Work out the finished part from the listing and answer in its coordinate system (mm). A direction names the side the tool comes from. Round coordinates to 2 decimals unless told otherwise and drop trailing zeros. Loops run counter-clockwise (first coordinate to the right, second up) from the corner with the lowest first, then second, coordinate; pieces in that order, holes last.
```python
from build123d import *

# Parameters (mm, degrees)
SKETCH1_W           = 20
SKETCH1_H           = 30
SKETCH1_R           = 2.65
BOSS_EXTRUDE1_DEPTH = 3
SKETCH2_W           = 20
SKETCH2_H           = 10
BOSS_EXTRUDE2_DEPTH = 3
SKETCH3_W           = 1.8
SKETCH3_H           = 10
BOSS_EXTRUDE3_DEPTH = 10
FILLET1_R           = 5
CUT_EXTRUDE1_REACH  = 29.78
SKETCH4_R           = 1.5
CHAMFER1_SIZE       = 2


with BuildPart() as part:
    # Sketch1 → Boss-Extrude1 (new body)
    with BuildSketch(Plane.XY):
        Rectangle(SKETCH1_W, SKETCH1_H)
        with Locations((0, -10)):
            Circle(SKETCH1_R, mode=Mode.SUBTRACT)
        Circle(SKETCH1_R, mode=Mode.SUBTRACT)
    extrude(amount=BOSS_EXTRUDE1_DEPTH)

    # Sketch2 → Boss-Extrude2 (add)
    with BuildSketch(Plane.XY.offset(3)):
        with Locations((0, 10)):
            Rectangle(SKETCH2_W, SKETCH2_H)
    extrude(amount=BOSS_EXTRUDE2_DEPTH)

    # Sketch3 → Boss-Extrude3 (add)
    with BuildSketch(Plane.XY.offset(6)):
        with Locations((-6.15, 10)):
            Rectangle(SKETCH3_W, SKETCH3_H)
        with Locations((6.15, 10)):
            Rectangle(SKETCH3_W, SKETCH3_H)
    extrude(amount=BOSS_EXTRUDE3_DEPTH)

    # Fillet1
    fillet1_edges = [part.edges().sort_by_distance(p)[0] for p in [
        (6.15, 5, 16),
        (-6.15, 5, 16),
        (6.15, 15, 16),
        (-6.15, 15, 16),
    ]]
    fillet(fillet1_edges, radius=FILLET1_R - 0.0001)  # a hair under: the kernel refuses the full size

    # Cut-Extrude1: up to this face of the body (flat: up to its plane)
    cut_extrude1_end = Plane(part.part.faces().sort_by_distance((7.05, 10, 10.533268934))[0])
    # Sketch4 → Cut-Extrude1 (cut, up to the picked face)
    with BuildSketch(Plane.ZY.offset(7.05), mode=Mode.PRIVATE) as cut_extrude1_sk1:
        with Locations(Location((11, 10, 0), (0, 0, 270))):
            Circle(SKETCH4_R)
    cut_extrude1_tool1 = split(extrude(cut_extrude1_sk1.sketch, amount=-CUT_EXTRUDE1_REACH, mode=Mode.PRIVATE), bisect_by=cut_extrude1_end, keep=Keep.BOTH, mode=Mode.PRIVATE)
    add(cut_extrude1_tool1.solids().sort_by(Axis((-7.05, 10, 11), (1, 0, 0)))[0], mode=Mode.SUBTRACT)

    # Chamfer1
    chamfer1_edges = [part.edges().sort_by_distance(p)[0] for p in [
        (-7.05, 10, 6),
        (7.05, 10, 6),
    ]]
    chamfer(chamfer1_edges, length=CHAMFER1_SIZE)


solid = part.part
```
1. Determine the mould class of faces 1 (the face through (-5.25, 8.8, 9.8)), 2 (the face through (0, 5, 5)), 3 (the face through (-0.57, -12.59, 1.48)) for opening direction Y: +Y half, -Y half, draft (parallel to the pull), parting line (faces both ways), or undercut.
Answer key:
face 1: draft
face 2: -Y half
face 3: undercut
2. Find section B-B (z = 6.75). Write down the section's boundary in (x, y).
Answer key:
outline: (-8.3, 5) - (-5.25, 5) - (-5.25, 15) - (-8.3, 15) - close; (5.25, 5) - (8.3, 5) - (8.3, 15) - (5.25, 15) - close
3. Which of the six approach directions +Z, -Z, +X, -X, +Y, -Y give full straight-line access (tool end or side, diameter ignored) to faces 4 (the face through (-7.05, 10, 13)), 5 (the face through (0, -5, 3)), 6 (the face through (5.25, 8.8, 9.8)), 7 (the face through (9.5, 10.1, 6))?
Answer key:
face 4: +Z, -X, +Y, -Y
face 5: +Z, +X, -X, -Y
face 6: +Z, +Y, -Y
face 7: +Z, +X, +Y, -Y
4. Find section D-D (z = 2.25). Write down the section's boundary in (x, y).
Answer key:
outline: (-10, -15) - (10, -15) - (10, 15) - (-10, 15) - close; hole circle Ø5.3 at (0, -10); hole circle Ø5.3 at (0, 0)
5. Find section A-A (y = -10). Write down the section's boundary in (x, z).
Answer key:
outline: (-10, 0) - (-2.65, 0) - (-2.65, 3) - (-10, 3) - close; (2.65, 0) - (10, 0) - (10, 3) - (2.65, 3) - close
6. Given pin 1 (6 mm diameter, centred on y = 11.5, z = 12, fed in from -X); pin 2 (2.5 mm diameter, centred on y = 8, z = 13, fed in from +X); pin 3 (1 mm diameter, centred on x = 7, z = 11.5, fed in from -Y); pin 4 (5 mm diameter, centred on y = -9, z = 3.5, fed in from +X), each flat-ended and moving along its own axis, determine where each tip first touches the part or whether it passes through.
Answer key:
pin 1: stops at x = -7.05
pin 2: stops at x = 7.05
pin 3: stops at y = 5
pin 4: stops at x = 10
7. Consider probe 1 along Y at (x, z) = (0, 0.6); probe 2 along X at (y, z) = (8.5, 13.75); probe 3 along Z at (x, y) = (5.85, 10). Determine where each line is inside the solid, lowest interval first.
Answer key:
probe 1: y = -15 to -12.65, -7.35 to -2.65, 2.65 to 15
probe 2: x = -7.05 to -5.25, 5.25 to 7.05
probe 3: z = 0 to 9.5, 12.5 to 16
8. Find section C-C (x = 0). Write down the section's boundary in (y, z), then the cut area to 3 significant figures.
Answer key:
outline: (-15, 0) - (-12.65, 0) - (-12.65, 3) - (-15, 3) - close; (-7.35, 0) - (-2.65, 0) - (-2.65, 3) - (-7.35, 3) - close; (2.65, 0) - (15, 0) - (15, 6) - (5, 6) - (5, 3) - (2.65, 3) - close
area: 88.2 mm2
